Check sheet for the drawn part. Datum: minimum x, y, z corner. Units: mm. A direction names the side the tool comes from. Round coordinates to 2 decimals unless told otherwise and drop trailing zeros. Write each loop counter-clockwise with the first axis right and the second up, starting at its lowest first coordinate (ties: lowest second). Pieces come first, ordered by that corner, then holes. Notation, with made-up numbers: (54, 61.5) -> (111, 61.5) arc R9 ccw to (111, 70.5) -> close; hole circle Ø10 at (59.5, 47.5). An arc over 180 degrees is marked (long way). Use a Markdown table: item, result.
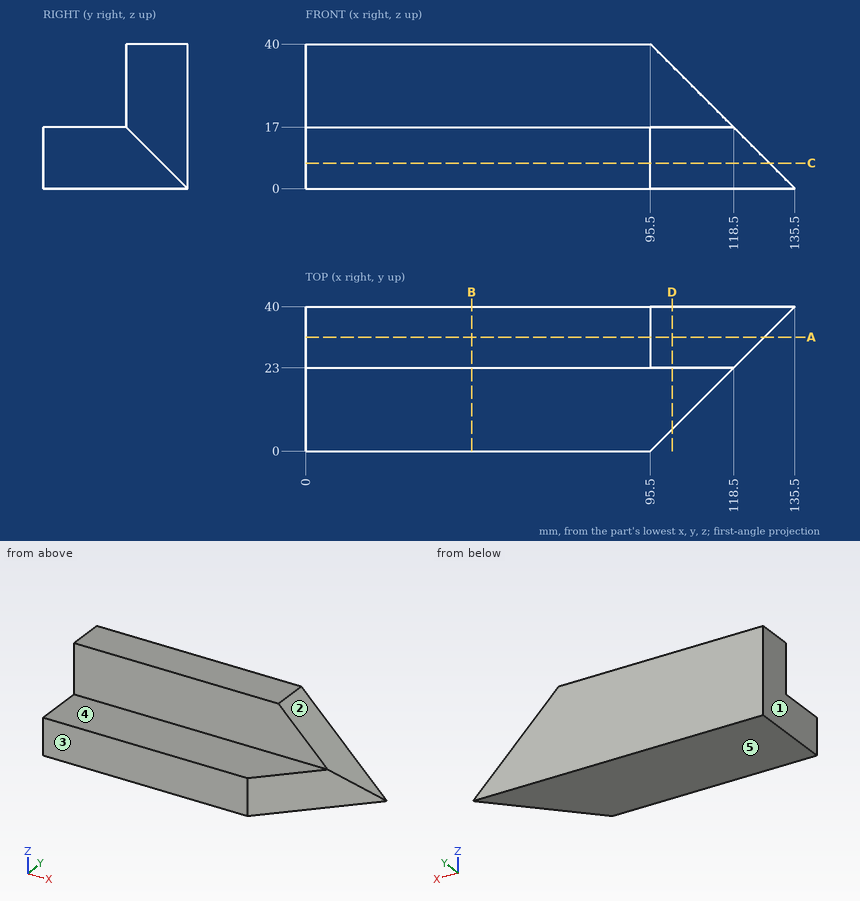
(1) Access from +Z, -Z, +X, -X, +Y, -Y to the whole of each face (thin tool, end or side, straight path). Record for the marked faces 4 and 5.
A:
| item | result |
|---|---|
| face 4 | +Z, +X, -X, -Y |
| face 5 | -Z, +X, -X, +Y, -Y |
(2) Thickness scan on line 1 (Y direction, x = 17.5, z = 32); line 2 (Z direction, x = 108.5, y = 16); line 3 (X direction, y = 37.5, z = 23). Record the ranges inside material, lowest first.
A:
| item | result |
|---|---|
| line 1 | y = 23 to 40 |
| line 2 | z = 0 to 17 |
| line 3 | x = 0 to 112.5 |
(3) Section check A-A on y = 31.5. Record the cut outline in (x, z), plus the area to 3 significant figures.
A:
| item | result |
|---|---|
| outline | (0, 0) -> (127, 0) -> (127, 8.5) -> (95.5, 40) -> (0, 40) -> close |
| area | 4,580 mm2 |
(4) Section check D-D on x = 101.5. Record the cut outline in (y, z).
A:
| item | result |
|---|---|
| outline | (6, 0) -> (40, 0) -> (40, 34) -> (23, 34) -> (23, 17) -> (6, 17) -> close |
(5) Section check C-C on z = 7. Record the cut outline in (x, y), plus the area to 3 significant figures.
A:
| item | result |
|---|---|
| outline | (0, 0) -> (95.5, 0) -> (128.5, 33) -> (128.5, 40) -> (0, 40) -> close |
| area | 4,600 mm2 |
(6) Gauge pin test, flat ends, axial feed: pin 1 Ø11.5 at (x, z) = (69.5, 23) entering from -Y; pin 2 Ø12 at (x, z) = (105, 15) entering from -Y; pin 3 Ø18.5 at (x, y) = (73, 14) entering from +Z. Record the tip position at first contact, or that the pin passes through.
A:
| item | result |
|---|---|
| pin 1 | stops at y = 23 |
| pin 2 | stops at y = 3.5 |
| pin 3 | stops at z = 40 |
(7) Section check B-B on x = 46. Record the cut outline in (y, z).
A:
| item | result |
|---|---|
| outline | (0, 0) -> (40, 0) -> (40, 40) -> (23, 40) -> (23, 17) -> (0, 17) -> close |
(8) Release check for a two-part mould opening along X. For the marked faces 1, 2 and 3 record: +X half, -X half, draft (parallel to the pull), parting line (faces both ways), or undercut.
A:
| item | result |
|---|---|
| face 1 | -X half |
| face 2 | +X half |
| face 3 | draft |
